Work out the finished part from the listing and answer in its coordinate system (mm). A direction names the side the tool comes from. Coordinates: 2 decimals unless noted, no trailing zeros. Loops run counter-clockwise (first coordinate to the right, second up) from the corner with the lowest first, then second, coordinate; pieces in that order, holes last. Notation, with made-up numbers: (13.5, -13) -> (18.5, -13) arc R25 cw to (18.5, 12) -> close; hole circle Ø8 at (38, -37.5). An arc over 180 degrees is marked (long way). Use a Markdown table: item, result.
from build123d import *

# Parameters (mm, degrees)
F0_R     = 6.604
F1_DEPTH = 25.4
F2_R     = 1.27
F5_DEPTH = 19.812


with BuildPart() as f1:
    # F0 (on Right) → F1 (new body)
    with BuildSketch(Plane.YZ):
        with BuildLine():
            Line((-44.9730095259, 19.512440572), (-60.2130095259, 19.512440572))
            Line((-60.2130095259, 19.512440572), (-60.2130095259, 10.6997340918))
            Line((-60.2130095259, 10.6997340918), (-10.535961017, 10.6997340918))
            Line((-10.535961017, 10.6997340918), (-10.535961017, -6.1869150959))
            Line((-10.535961017, -6.1869150959), (-29.7518018633, -6.1869150959))
            Line((-29.7518018633, -6.1869150959), (-29.7518018633, -17.9784540087))
            Line((-29.7518018633, -17.9784540087), (0, -17.9784540087))
            Line((0, -17.9784540087), (29.7518018633, -17.9784540087))
            Line((29.7518018633, -17.9784540087), (29.7518018633, -6.1869150959))
            Line((29.7518018633, -6.1869150959), (10.535961017, -6.1869150959))
            Line((10.535961017, -6.1869150959), (10.535961017, 10.6997340918))
            Line((10.535961017, 10.6997340918), (60.2130095259, 10.6997340918))
            Line((60.2130095259, 10.6997340918), (60.2130095259, 19.512440572))
            Line((60.2130095259, 19.512440572), (44.9730095259, 19.512440572))
            Line((44.9730095259, 19.512440572), (10.1265067253, 36.4959567288))
            ThreePointArc((10.1265067253, 36.4959567288), (10.587250916, 34.7297929897), (10.7423247602, 32.911119939))
            ThreePointArc((10.7423247602, 32.911119939), (-1.5527814637, 22.281940137), (-10.2926816094, 35.9846130792))
            Line((-10.2926816094, 35.9846130792), (-44.9730095259, 19.512440572))
        make_face()
        with BuildLine():
            ThreePointArc((10.1265067253, 36.4959567288), (-0.2686387048, 43.6497954823), (-10.2926816094, 35.9846130792))
            ThreePointArc((-10.2926816094, 35.9846130792), (-1.5527814637, 22.281940137), (10.7423247602, 32.911119939))
            ThreePointArc((10.7423247602, 32.911119939), (10.587250916, 34.7297929897), (10.1265067253, 36.4959567288))
        make_face()
        with Locations((0.0002825399, 32.911119939)):
            Circle(F0_R, mode=Mode.SUBTRACT)
    extrude(amount=F1_DEPTH)

    # F2
    f2_edges = [f1.edges().sort_by_distance(p)[0] for p in [
        (25.4, -27.632846, 27.748527),
        (25.4, -0.268639, 43.649795),
        (25.4, 27.549758, 28.004199),
        (25.4, 52.59301, 19.512441),
        (25.4, -52.59301, 19.512441),
        (12.7, -44.97301, 19.512441),
        (12.7, -60.21301, 19.512441),
        (0, -52.59301, 19.512441),
        (0, -27.632846, 27.748527),
        (0, -0.268639, 43.649795),
        (0, 27.549758, 28.004199),
        (0, 52.59301, 19.512441),
        (12.7, 60.21301, 19.512441),
        (12.7, 44.97301, 19.512441),
        (12.7, -10.292682, 35.984613),
        (12.7, 10.126507, 36.495957),
    ]]
    fillet(f2_edges, radius=F2_R)

    # F4 (on offset) → F5 (join)
    with BuildSketch(Plane.YZ.offset(44.958)):
        Polygon((-60.2130095259, 42.8991168737), (-60.2130095259, 18.242440572), (-60.2130095259, 10.6997340918), (60.2849709341, 10.6997340918), (60.4153525641, 42.8991168737), align=None)
    extrude(amount=-F5_DEPTH)


solid = f1.part
Q1. Section A-A on x = 9 is taken. Determine the outline of the cut face in (y, z), and give its area (3 significant figures).
Solved:
| item | result |
|---|---|
| outline | (-60.21, 10.7) -> (-10.54, 10.7) -> (-10.54, -6.19) -> (-29.75, -6.19) -> (-29.75, -17.98) -> (29.75, -17.98) -> (29.75, -6.19) -> (10.54, -6.19) -> (10.54, 10.7) -> (60.21, 10.7) -> (60.21, 18.24) arc R1.27 ccw to (58.94, 19.51) -> (45.27, 19.51) arc R1.27 cw to (44.71, 19.64) -> (10.58, 36.28) arc R1.27 cw to (9.96, 36.94) arc R10.74 ccw to (-10.13, 36.48) arc R1.27 cw to (-10.79, 35.75) -> (-44.71, 19.64) arc R1.27 cw to (-45.26, 19.51) -> (-58.94, 19.51) arc R1.27 ccw to (-60.21, 18.24) -> close; hole circle Ø13.21 at (0, 32.91) |
| area | 3,020 mm² |
Q2. Section C-C on x = 39 is taken. Determine the outline of the cut face in (y, z), and give its area (3 significant figures).
Solved:
| item | result |
|---|---|
| outline | (-60.21, 10.7) -> (60.28, 10.7) -> (60.42, 42.9) -> (-60.21, 42.9) -> close |
| area | 3,880 mm² |
Q3. For faces 1 (the flat face through (12, 60.213, 14)), 2 (the flat face through (25.146, 0, 33)), 3 (the flat face through (13, 20, -6.187)), determine the directions among +Z, -Z, +X, -X, +Y, -Y from which every point of the face is accessible in a straight line to the end or side of a thin tool.
Solved:
| item | result |
|---|---|
| face 1 | +Z, -Z, -X, +Y |
| face 2 | -X |
| face 3 | +X, -X, +Y |
Q4. Determine the mould class of faces 4 (the flat face through (35, 1, 42.899)), 5 (the cylindrical face through (12.397, -1.431, 26.464)), 6 (the flat face through (13, 29.752, -12)) for opening direction Y: pulls with the +Y half, pulls with the -Y half, needs draft (parallel to the pull), parting line crosses it, or undercut.
Solved:
| item | result |
|---|---|
| face 4 | needs draft |
| face 5 | undercut |
| face 6 | pulls with the +Y half |
Q5. Section B-B on z = 2 is taken. Determine the outline of the cut face in (x, y), and give its area (3 significant figures).
Solved:
| item | result |
|---|---|
| outline | (0, -10.54) -> (25.4, -10.54) -> (25.4, 10.54) -> (0, 10.54) -> close |
| area | 535 mm² |
Q6. Consider line 1 (Y direction, x = 12.5, z = -7); line 2 (Z direction, x = 32, y = -4.5); line 3 (Z direction, x = 6, y = 31). Determine where each line is inside the solid, lowest interval first. Write a range as [from, to].
Solved:
| item | result |
|---|---|
| line 1 | [-29.75, 29.75] |
| line 2 | [10.7, 42.9] |
| line 3 | [10.7, 26.32] |
Q7. Given pin 1 Ø4 at (x, y) = (9.5, -50) entering from +Z; pin 2 Ø9.5 at (x, y) = (6.5, 19.5) entering from +Z; pin 3 Ø8 at (x, y) = (27, 24) entering from +Z, each flat-ended and moving along its own axis, determine where each tip first touches the part or whether it passes through.
Solved:
| item | result |
|---|---|
| pin 1 | z = 19.51 |
| pin 2 | z = 34.24 |
| pin 3 | z = 42.9 |
